from build123d import *

# Parameters (mm, degrees)
F0_W     = 1219.2
F0_H     = 1219.2
F1_DEPTH = 12.7
F3_DEPTH = 12.701
F5_DEPTH = 12.701
F6_W     = 6.35
F6_H     = 44.45
F6_W_2   = 44.45
F6_H_2   = 6.35
F7_DEPTH = 12.701


with BuildPart() as f1:
    # F0 (on Top) → F1 (new body)
    with BuildSketch(Plane.XY):
        with Locations((609.6, 609.6)):
            Rectangle(F0_W, F0_H)
    extrude(amount=F1_DEPTH)

    # F2 (on face) → F3 (cut, through all)
    with BuildSketch(Plane(origin=(0, 0, 0), x_dir=(1, 0, 0), z_dir=(0, 0, -1))):
        Polygon((50.8, -254), (0, -203.2), (0, -1219.2), (1016, -1219.2), (965.2, -1168.4), (152.4, -1066.8), align=None)
    extrude(amount=-F3_DEPTH, mode=Mode.SUBTRACT)

    # F4 (on face) → F5 (cut, through all)
    with BuildSketch(Plane(origin=(0, 0, 0), x_dir=(1, 0, 0), z_dir=(0, 0, -1))):
        Polygon((254, -50.8), (1066.8, -152.4), (1168.4, -965.2), (1219.2, -1016), (1219.2, 0), (203.2, 0), align=None)
    extrude(amount=-F5_DEPTH, mode=Mode.SUBTRACT)

    # F6 (on face) → F7 (cut, through all)
    with BuildSketch(Plane.XY.offset(12.7)):
        with Locations((606.425, 581.025)):
            Rectangle(F6_W, F6_H)
        with Locations((612.775, 581.025)):
            Rectangle(F6_W, F6_H)
        with Locations((581.025, 612.775)):
            Rectangle(F6_W_2, F6_H_2)
        with Locations((581.025, 606.425)):
            Rectangle(F6_W_2, F6_H_2)
        with Locations((638.175, 612.775)):
            Rectangle(F6_W_2, F6_H_2)
        with Locations((638.175, 606.425)):
            Rectangle(F6_W_2, F6_H_2)
        with Locations((606.425, 612.775)):
            Rectangle(F6_W, F6_H_2)
        with Locations((612.775, 612.775)):
            Rectangle(F6_W, F6_H_2)
        with Locations((606.425, 606.425)):
            Rectangle(F6_W, F6_H_2)
        with Locations((612.775, 606.425)):
            Rectangle(F6_W, F6_H_2)
        with Locations((606.425, 638.175)):
            Rectangle(F6_W, F6_H)
        with Locations((612.775, 638.175)):
            Rectangle(F6_W, F6_H)
    extrude(amount=-F7_DEPTH, mode=Mode.SUBTRACT)


solid = f1.part
Geometry check sheet. Reference: the model listing, model coordinates, mm. Give positions to 0.01 mm unless a question says otherwise; leave off trailing zeros. Order: outer loops, then holes, each group sorted by start corner. A loop starts at its lowest first (then second) coordinate and runs counter-clockwise, first axis right, second up. Notation, with made-up numbers: (70.25, 83) - (89.25, 83) arc R17 ccw to (89.25, 91) - close; hole circle Ø6 at (8, 10.25). An arc over 180 degrees is marked (long way). Answer as a JSON object with one key per item and string values.
(1) Cross-section at B-B (x = 816). Record the cut outline in (y, z).
Report:
{"outline": "(121.05, 0) - (1149.75, 0) - (1149.75, 12.7) - (121.05, 12.7) - close"}
(2) Depth check by flat-ended pin: pin 1 Ø4 at (y, z) = (630.5, 8.5) entering from +X; pin 2 Ø4 at (x, z) = (639, 9.5) entering from +Y (3 decimals); pin 3 Ø5 at (y, z) = (672.5, 6.5) entering from -X. Enter the tip coordinate at first touch or a pass-through.
Report:
{"pin 1": "x = 1126.81", "pin 2": "y = 1127.875", "pin 3": "x = 102.8"}
(3) Cross-section at A-A (z = 5). Record the cut outline in (x, y), then the cut area to 3 significant figures.
Report:
{"outline": "(0, 0) - (203.2, 0) - (254, 50.8) - (1066.8, 152.4) - (1168.4, 965.2) - (1219.2, 1016) - (1219.2, 1219.2) - (1016, 1219.2) - (965.2, 1168.4) - (152.4, 1066.8) - (50.8, 254) - (0, 203.2) - close; hole (558.8, 603.25) - (603.25, 603.25) - (603.25, 558.8) - (615.95, 558.8) - (615.95, 603.25) - (660.4, 603.25) - (660.4, 615.95) - (615.95, 615.95) - (615.95, 660.4) - (603.25, 660.4) - (603.25, 615.95) - (558.8, 615.95) - close", "area": "1,100,000 mm^2"}
(4) Material ranges on line 1 (Y direction, x = 656.5, z = 10.25); line 2 (X direction, y = 244.5, z = 10); line 3 (Y direction, x = 881, z = 8.5) (3 decimals), recorded low to high.
Report:
{"line 1": "101.11 to 603.25, 615.95 to 1129.81", "line 2": "41.3 to 1078.31", "line 3": "129.175 to 1157.875"}
(5) Cross-section at C-C (y = 1125.5). Record the cut outline in (x, z).
Report:
{"outline": "(622, 0) - (1219.2, 0) - (1219.2, 12.7) - (622, 12.7) - close"}
